Model file for the job. Use its own axes, mm. Round coordinates to 2 decimals unless told otherwise and drop trailing zeros. Order: outer loops, then holes, each group sorted by start corner. A loop starts at its lowest first (then second) coordinate and runs counter-clockwise, first axis right, second up. Notation, with made-up numbers: (66.25, 8) -> (118.25, 8) arc R18 cw to (118.25, 26) -> close; hole circle Ø8 at (32.25, -39). An arc over 180 degrees is marked (long way). Put each result on its own line as item: value. Start each with the question number.
Q1. Cut at C-C, the plane y = -5.25. List the corners of the cut face in (x, z), and give its area (3 significant figures).
Q2. Probe L1, parallel to Z at x = 0, y = -18.5; L2, parallel to Z at x = -1.5, y = -9.5; L3, parallel to Z at x = 6, y = -3. List the from-to ranges inside material, lowest first.
Q3. Pull direction X, two halves, no side cores. Call faces 1 (the face through (-0.83, -12.88, -29.12)), 2 (the face through (-29.206, -12.878, 0.168)), 3 (the face through (-1, 0, -11)), 4 (the face through (-6.613, -12.522, 50.366)): released by +X, released by -X, zero draft, split by the parting line, or undercut.
Q4. Cut at B-B, the plane x = -27. List the corners of the cut face in (y, z).
Q5. Cut at D-D, the plane z = 25.4. List the corners of the cut face in (x, y), and give its area (3 significant figures).
Q6. Flat gauge pins, fed straight in: P1, Ø5, axis at y = -11, z = -30.5, coming from the +X side (3 decimals); P2, Ø6, axis at y = -21, z = -8.5, coming from the -X side; P3, Ø12, axis at y = -21.5, z = -7.5, coming from the +X side. Where does each tip first touch, or does it go through?
Q7. Cut at A-A, the plane z = 0. List the corners of the cut face in (x, y), and give its area (3 significant figures).
from build123d import *

# Parameters (mm, degrees)
F0_R     = 50.798489
F1_DEPTH = 25.4
F2_R     = 8.018055
F3_DEPTH = 88.392
F4_R     = 3.81
F6_DEPTH = 25.4


with BuildPart() as f1:
    # F0 (on Front) → F1 (new body)
    with BuildSketch(Plane.XZ):
        Circle(F0_R)
    extrude(amount=F1_DEPTH)

    # F2 (on face) → F3 (cut)
    with BuildSketch(Plane.XZ.offset(25.4)):
        Circle(F2_R)
    extrude(amount=-F3_DEPTH, mode=Mode.SUBTRACT)

    # F4 (on face) → F6 (cut)
    with BuildSketch(Plane.XZ.offset(25.4)):
        with Locations((0, 25.4)):
            Circle(F4_R)
        with Locations((-25.4, 0)):
            Circle(F4_R)
        with Locations((0, -25.4)):
            Circle(F4_R)
        with Locations((25.4, 0)):
            Circle(F4_R)
    extrude(amount=-F6_DEPTH, mode=Mode.SUBTRACT)


solid = f1.part
Ans:
1. outline: circle Ø101.6 at (0, 0); hole circle Ø7.62 at (-25.4, 0); hole circle Ø16.04 at (0, 0); hole circle Ø7.62 at (0, -25.4); hole circle Ø7.62 at (0, 25.4); hole circle Ø7.62 at (25.4, 0)
1. area: 7,720 mm^2
2. L1: z = -50.8 to -29.21, -21.59 to -8.02, 8.02 to 21.59, 29.21 to 50.8
2. L2: z = -50.78 to -28.9, -21.9 to -7.88, 7.88 to 21.9, 28.9 to 50.78
2. L3: z = -50.44 to -5.32, 5.32 to 50.44
3. face 1: undercut
3. face 2: undercut
3. face 3: zero draft
3. face 4: split by the parting line
4. outline: (-25.4, -43.03) -> (0, -43.03) -> (0, -3.46) -> (-25.4, -3.46) -> close; (-25.4, 3.46) -> (0, 3.46) -> (0, 43.03) -> (-25.4, 43.03) -> close
5. outline: (-43.99, -25.4) -> (-3.81, -25.4) -> (-3.81, 0) -> (-43.99, 0) -> close; (3.81, -25.4) -> (43.99, -25.4) -> (43.99, 0) -> (3.81, 0) -> close
5. area: 2,040 mm^2
6. P1: stops at x = 42.385
6. P2: stops at x = -50.5
6. P3: stops at x = 50.78
7. outline: (-50.8, -25.4) -> (-29.21, -25.4) -> (-29.21, 0) -> (-50.8, 0) -> close; (-21.59, -25.4) -> (-8.02, -25.4) -> (-8.02, 0) -> (-21.59, 0) -> close; (8.02, -25.4) -> (21.59, -25.4) -> (21.59, 0) -> (8.02, 0) -> close; (29.21, -25.4) -> (50.8, -25.4) -> (50.8, 0) -> (29.21, 0) -> close
7. area: 1,790 mm^2
